Read the model definition and answer for the solid it produces. Units are mm, in the model's axes. A direction names the side the tool comes from. Round coordinates to 2 decimals unless told otherwise and drop trailing zeros. Order: outer loops, then holes, each group sorted by start corner. A loop starts at its lowest first (then second) coordinate and runs counter-clockwise, first axis right, second up. Notation, with made-up numbers: (11.25, 70.5) -> (65.25, 70.5) arc R15 ccw to (65.25, 95.5) -> close; hole circle Ø8 at (-31.75, 14). An arc over 180 degrees is marked (long way). Use a Markdown table: item, result. Add a question column.
1. Section D-D, the plane y = -53 is taken. Give the vertices of the cut face in (x, z), then the cut area to 3 significant figures.
2. Given pin 1 (11 mm diameter, centred on y = -176.5, z = 22.5, fed in from -X); pin 2 (8 mm diameter, centred on x = -5, y = -41, fed in from +Z); pin 3 (4 mm diameter, centred on y = -82, z = 4.5, fed in from +X); pin 4 (2 mm diameter, centred on x = -0.5, z = 1.5, fed in from +Y), each flat-ended and moving along its own axis, determine where each tip first touches the part or whether it passes through.
3. For faces 1 (the face through (0, -5.754, 5)), 2 (the face through (5, -173, 19)), 3 (the face through (0, -3, 0)), 4 (the face through (0, -102, 2.5)), determine the directions among +Z, -Z, +X, -X, +Y, -Y from which every point of the face is accessible in a straight line to the end or side of a thin tool.
4. Consider L1, parallel to Y at x = 0, z = 0.9 (3 decimals); L2, parallel to X at y = 0, z = 0.55; L3, parallel to Z at x = 1, y = -176. Determine where each line is inside the solid, lowest interval first. Write a range as [from, to].
5. Section C-C, the plane z = -4 is taken. Give the vertices of the cut face in (x, y).
6. Section B-B, the plane y = -8 is taken. Give the vertices of the cut face in (x, z), then the cut area to 3 significant figures.
7. The mould has two halves that part along X. Classify faces 5 (the face through (5, -82, 5)), 6 (the face through (0.07, 2.1, 1.23)), 7 (the face through (-5, -97, 5)): +X half, -X half, draft (parallel to the pull), parting line (faces both ways), or undercut.
8. Section A-A, the plane x = 8.5 is taken. Give the vertices of the cut face in (y, z), then the cut area to 3 significant figures.
```python
from build123d import *

# Parameters (mm, degrees)
SKETCH2_R           = 12.5
BOSS_EXTRUDE1_DEPTH = 2.5
BOSS_EXTRUDE2_DEPTH = 5
BOSS_EXTRUDE3_DEPTH = 15
SKETCH9_W           = 5
SKETCH9_H           = 25
BOSS_EXTRUDE4_DEPTH = 10
CUT_EXTRUDE1_DEPTH  = 142


with BuildPart() as part:
    # Sketch2 → Boss-Extrude1 (new body)
    with BuildSketch(Plane.XY):
        Circle(SKETCH2_R)
        with BuildLine():
            ThreePointArc((1.389019438, -1.575), (0, 2.1), (-1.389019438, -1.575))
            Line((-1.389019438, -1.575), (0, -1.575))
            Line((0, -1.575), (1.389019438, -1.575))
        make_face(mode=Mode.SUBTRACT)
    extrude(amount=BOSS_EXTRUDE1_DEPTH)

    # Sketch4 → Boss-Extrude2 (add)
    with BuildSketch(Plane.XY.offset(2.5)):
        Polygon((-5, -165.75443039), (5, -165.75443039), (5, -5.75443039), (0, -5.75443039), (-5, -5.75443039), align=None)
    extrude(amount=BOSS_EXTRUDE2_DEPTH)

    # Sketch5 → Boss-Extrude3 (add)
    with BuildSketch(Plane(origin=(5, 0, 0), x_dir=(0, 0, -1), z_dir=(1, 0, 0))):
        Polygon((20, -155.75443039), (-5, -155.75443039), (-30, -155.75443039), (-30, -190.75443039), (-5, -190.75443039), (20, -190.75443039), align=None)
    extrude(amount=BOSS_EXTRUDE3_DEPTH)

    # Sketch9 → Boss-Extrude4 (add)
    with BuildSketch(Plane.ZY.offset(5)):
        with Locations((5, -178.25443039)):
            Rectangle(SKETCH9_W, SKETCH9_H)
    extrude(amount=-BOSS_EXTRUDE4_DEPTH)

    # Sketch6 → Cut-Extrude1 (cut)
    with BuildSketch(Plane(origin=(0, 0, -20), x_dir=(-1, 0, 0), z_dir=(0, 0, -1))):
        with BuildLine():
            Line((-5, -155.75443039), (-20, -155.75443039))
            Line((-20, -155.75443039), (-20, -190.75443039))
            ThreePointArc((-20, -190.75443039), (-8.963631912, -174.770016714), (-5, -155.75443039))
        make_face()
    extrude(amount=-CUT_EXTRUDE1_DEPTH, mode=Mode.SUBTRACT)


solid = part.part
```
Verdict:
| question | item | result |
|---|---|---|
| 1 | outline | (-5, 2.5) -> (5, 2.5) -> (5, 7.5) -> (-5, 7.5) -> close |
| 1 | area | 50.0 mm2 |
| 2 | pin 1 | stops at x = 5 |
| 2 | pin 2 | stops at z = 7.5 |
| 2 | pin 3 | stops at x = 5 |
| 2 | pin 4 | stops at y = 12.5 |
| 3 | face 1 | +Z, +X, -X, +Y |
| 3 | face 2 | +Z, -X, +Y, -Y |
| 3 | face 3 | -Z, +X, -X, +Y |
| 3 | face 4 | -Z, -X, -Y |
| 4 | L1 | y = [-12.5, -1.575], [2.1, 12.5] |
| 4 | L2 | x = [-12.5, -2.1], [2.1, 12.5] |
| 4 | L3 | z = [2.5, 7.5] |
| 5 | outline | (5, -190.75) -> (20, -190.75) arc R49.03 cw to (5, -155.75) -> close |
| 6 | outline | (-9.6, 0) -> (9.6, 0) -> (9.6, 2.5) -> (5, 2.5) -> (5, 7.5) -> (-5, 7.5) -> (-5, 2.5) -> (-9.6, 2.5) -> close |
| 6 | area | 98.0 mm2 |
| 7 | face 5 | +X half |
| 7 | face 6 | undercut |
| 7 | face 7 | -X half |
| 8 | outline | (-190.75, -20) -> (-173.65, -20) -> (-173.65, 30) -> (-190.75, 30) -> close; (-9.17, 0) -> (9.17, 0) -> (9.17, 2.5) -> (-9.17, 2.5) -> close |
| 8 | area | 901 mm2 |
